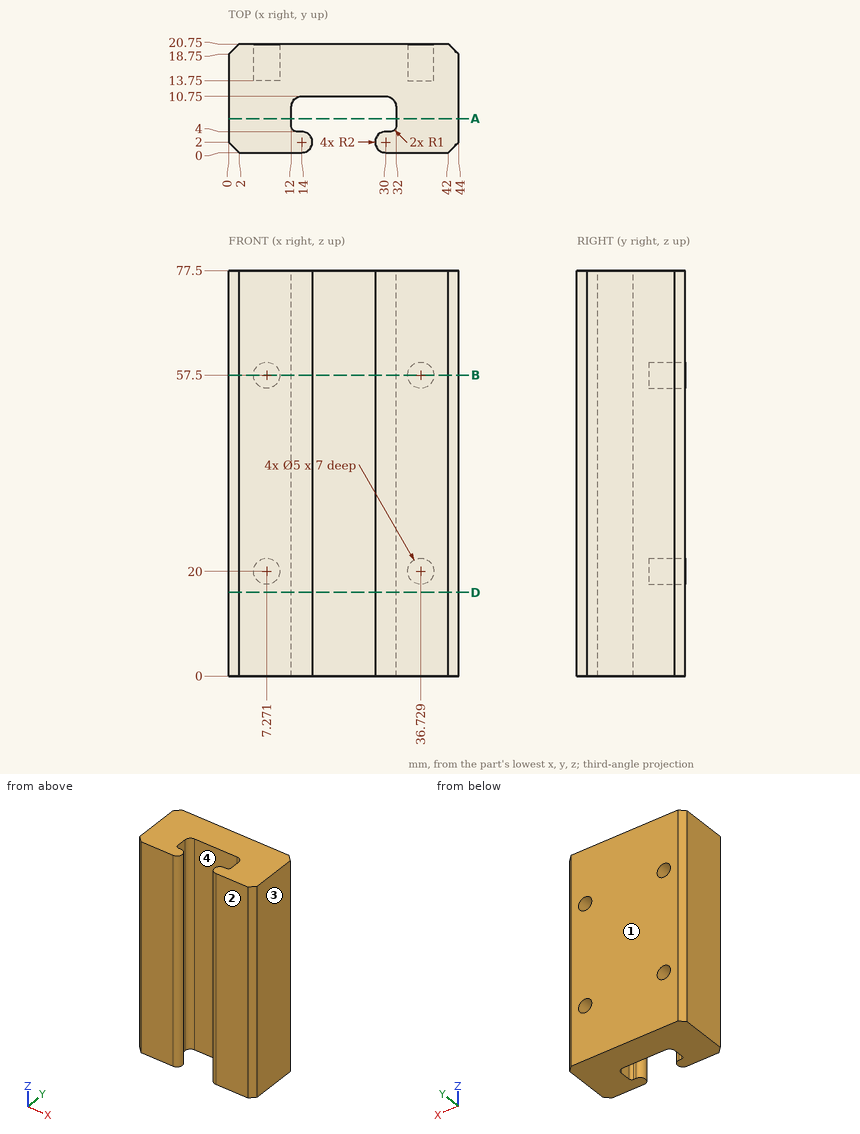
Print and shaded views of the part. All mm, measured from the part's lowest x, y and z. Coordinates: 2 decimals unless noted, no trailing zeros. Write each loop counter-clockwise with the first axis right and the second up, starting at its lowest first coordinate (ties: lowest second). Pieces come first, ordered by that corner, then holes. Notation, with made-up numbers: (70, 61.5) - (126, 61.5) arc R28 cw to (126, 92.5) - close; hole circle Ø9 at (67, 86). An arc over 180 degrees is marked (long way). One line per question, with ' | ' between items. Start each with the question number.
Q1. Cut at B-B, the plane z = 57.5. List the corners of the cut face in (x, y).
Q2. Pin check, flat tips, straight feed: pin 1 (1 mm diameter, centred on x = 16.5, y = 3, fed in from -Z); pin 2 (1.5 mm diameter, centred on x = 7, z = 19.5, fed in from +Y). Stop position of each tip, or through.
Q3. Drill centre lines: line 1 (Z direction, x = 7.5, y = 18); line 2 (X direction, y = 8.5, z = 66.5); line 3 (Z direction, x = 38, y = 15). Where is each one in solid material? Low to high. Write a range as [from, to].
Q4. Cut at A-A, the plane y = 6.5. List the corners of the cut face in (x, z).
Q5. Pull direction Y, two halves, no side cores. Call the marked faces 1, 2, 3 and 4: pulls with the +Y half, pulls with the -Y half, needs draft (parallel to the pull), parting line crosses it, or undercut.
Q6. Cut at D-D, the plane z = 16. List the corners of the cut face in (x, y).
Answer below:
1) outline: (0, 2) - (2, 0) - (14, 0) arc R2 ccw to (14, 4) - (13, 4) arc R1 cw to (12, 5) - (12, 8.75) arc R2 cw to (14, 10.75) - (30, 10.75) arc R2 cw to (32, 8.75) - (32, 5) arc R1 cw to (31, 4) - (30, 4) arc R2 ccw to (30, 0) - (42, 0) - (44, 2) - (44, 18.75) - (42, 20.75) - (39.23, 20.75) - (39.23, 13.75) - (34.23, 13.75) - (34.23, 20.75) - (9.77, 20.75) - (9.77, 13.75) - (4.77, 13.75) - (4.77, 20.75) - (2, 20.75) - (0, 18.75) - close
2) pin 1: through | pin 2: y = 13.75
3) line 1: [0, 17.51], [22.49, 55.01], [59.99, 77.5] | line 2: [0, 12], [32, 44] | line 3: [0, 17.85], [22.15, 55.35], [59.65, 77.5]
4) outline: (0, 0) - (12, 0) - (12, 77.5) - (0, 77.5) - close; (32, 0) - (44, 0) - (44, 77.5) - (32, 77.5) - close
5) face 1: pulls with the +Y half | face 2: pulls with the -Y half | face 3: needs draft | face 4: undercut
6) outline: (0, 2) - (2, 0) - (14, 0) arc R2 ccw to (14, 4) - (13, 4) arc R1 cw to (12, 5) - (12, 8.75) arc R2 cw to (14, 10.75) - (30, 10.75) arc R2 cw to (32, 8.75) - (32, 5) arc R1 cw to (31, 4) - (30, 4) arc R2 ccw to (30, 0) - (42, 0) - (44, 2) - (44, 18.75) - (42, 20.75) - (2, 20.75) - (0, 18.75) - close
